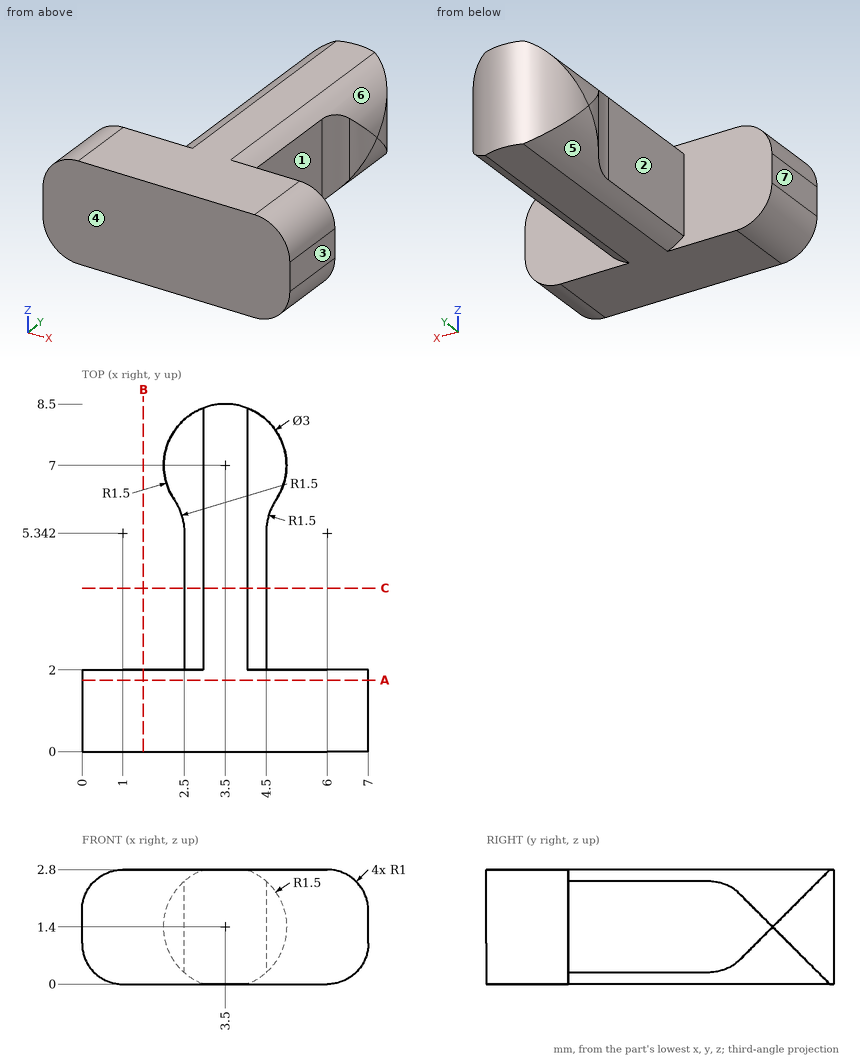
Part print with two shaded views. Sizes in mm from the minimum x, y, z corner. A direction names the side the tool comes from. Coordinates: 2 decimals unless noted, no trailing zeros. Write each loop counter-clockwise with the first axis right and the second up, starting at its lowest first coordinate (ties: lowest second). Pieces come first, ordered by that corner, then holes. Notation, with made-up numbers: (68.5, 14.5) - (97.5, 14.5) arc R28 cw to (97.5, 43.5) - close; hole circle Ø6 at (29, 18.25). An arc over 180 degrees is marked (long way). Use a Markdown table: item, result. Add a question column.
Item 1: 3-axis set-ups, long thin cutter, end or side, ignore diameter. For the marked faces 5, 6 and 7: which of +Z, -Z, +X, -X, +Y, -Y reach the whole face in a straight line?
Item 2: Band-saw the part on B-B, the plane x = 1.5. Write the cut outline in (y, z).
Item 3: Two-plate mould, pull along Y, no slides. Class the marked faces 1, 2, 3 and 4: pulls with the +Y half, pulls with the -Y half, needs draft (parallel to the pull), parting line crosses it, or undercut.
Item 4: Drill centre lines: line 1 along Y through (x, z) = (1, 0.65); line 2 along X through (y, z) = (4.5, 1.1); line 3 along X through (y, z) = (1.5, 0.8). Where is each one in solid material? Low to high.
Item 5: Band-saw the part on A-A, the plane y = 1.75. Write the cut outline in (x, z).
Item 6: Drop a flat-ended pin along its axis: pin 1 (1.5 mm diameter, centred on y = 3, z = 2, fed in from +X). Give the stop position or say it passes through.
Item 7: Band-saw the part on C-C, the plane y = 4. Write the cut outline in (x, z).
A:
| question | item | result |
|---|---|---|
| 1 | face 5 | -Z, -X, +Y |
| 1 | face 6 | +Z, +X, +Y |
| 1 | face 7 | +Z, -Z, -X, +Y, -Y |
| 2 | outline | (0, 0) - (2, 0) - (2, 2.8) - (0, 2.8) - close |
| 3 | face 1 | undercut |
| 3 | face 2 | undercut |
| 3 | face 3 | needs draft |
| 3 | face 4 | pulls with the -Y half |
| 4 | line 1 | y = 0 to 2 |
| 4 | line 2 | x = 2.5 to 4.5 |
| 4 | line 3 | x = 0.02 to 6.98 |
| 5 | outline | (0, 1) arc R1 ccw to (1, 0) - (6, 0) arc R1 ccw to (7, 1) - (7, 1.8) arc R1 ccw to (6, 2.8) - (1, 2.8) arc R1 ccw to (0, 1.8) - close |
| 6 | pin 1 | stops at x = 4.5 |
| 7 | outline | (2.5, 0.28) arc R1.5 ccw to (2.96, 0) - (4.04, 0) arc R1.5 ccw to (4.5, 0.28) - (4.5, 2.52) arc R1.5 ccw to (4.04, 2.8) - (2.96, 2.8) arc R1.5 ccw to (2.5, 2.52) - close |
